Could you check a few things on this model? Use its own coordinates, in mm. Give positions to 0.01 mm unless a question says otherwise; leave off trailing zeros. Order: outer loops, then holes, each group sorted by start corner. A loop starts at its lowest first (then second) coordinate and runs counter-clockwise, first axis right, second up. Notation, with made-up numbers: M 65.25,86.5 L 107.25,86.5 A21 ccw 107.25,111.5 Z; hole C -39.5,22 d10. An arc over 180 degrees is marked long. Use a Markdown table: item, result. Add a question column.
Item 1: If I drill on L1, parallel to Y at x = 45, z = 3.3; L2, parallel to Y at x = 32, z = 4.35; L3, parallel to Y at x = -43.5, z = 3.6, over which ranges is the centre line in solid material (lowest first)? Write a range as from..to.
Item 2: Suppose I cut it at A-A on x = -25.5. Write out the boundary of the cut face in (y, z).
Item 3: Suppose I cut it at B-B on z = 4.2. Write out the boundary of the cut face in (x, y).
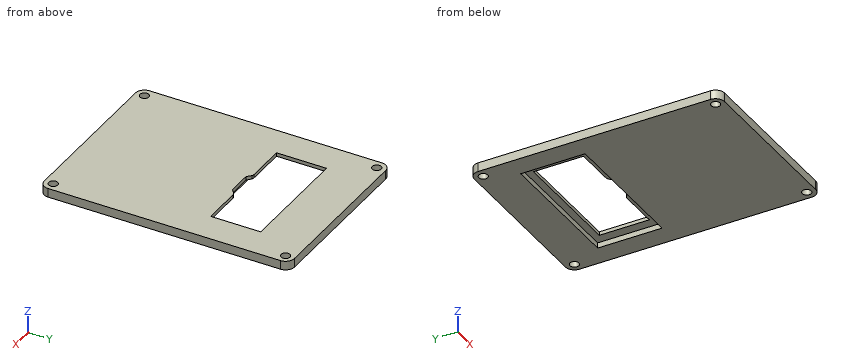
from build123d import *

# Parameters (mm, degrees)
SKETCH1_R           = 2.5
BOSS_EXTRUDE1_DEPTH = 5
CUT_EXTRUDE1_DEPTH  = 5
SKETCH2_4_W         = 76
SKETCH2_4_H         = 36
CUT_EXTRUDE2_DEPTH  = 3


with BuildPart() as part:
    # Sketch1 → Boss-Extrude1 (new body)
    with BuildSketch(Plane.XY):
        with BuildLine():
            Line((-45, 70), (45, 70))
            ThreePointArc((45, 70), (48.535533906, 68.535533906), (50, 65))
            Line((50, 65), (50, -65))
            ThreePointArc((50, -65), (48.535533906, -68.535533906), (45, -70))
            Line((45, -70), (-45, -70))
            ThreePointArc((-45, -70), (-48.535533906, -68.535533906), (-50, -65))
            Line((-50, -65), (-50, 65))
            ThreePointArc((-50, 65), (-48.535533906, 68.535533906), (-45, 70))
        make_face()
        with Locations((-45, 65)):
            Circle(SKETCH1_R, mode=Mode.SUBTRACT)
        with Locations((45, 65)):
            Circle(SKETCH1_R, mode=Mode.SUBTRACT)
        with Locations((45, -65)):
            Circle(SKETCH1_R, mode=Mode.SUBTRACT)
        with Locations((-45, -65)):
            Circle(SKETCH1_R, mode=Mode.SUBTRACT)
    extrude(amount=BOSS_EXTRUDE1_DEPTH)

    # Sketch2 → Cut-Extrude1 (cut)
    with BuildSketch(Plane(origin=(0, 0, 0), x_dir=(-1, 0, 0), z_dir=(0, 0, -1))):
        with BuildLine():
            Line((-8.935788795, 15.50990671), (-6.621919354, 13.5))
            Line((-6.621919354, 13.5), (6.621919354, 13.5))
            Line((6.621919354, 13.5), (8.935788795, 15.50990671))
            ThreePointArc((8.935788795, 15.50990671), (9.547279148, 15.873474502), (10.247345781, 16))
            Line((10.247345781, 16), (32.5, 16))
            Line((32.5, 16), (32.5, 44))
            Line((32.5, 44), (-32.5, 44))
            Line((-32.5, 44), (-32.5, 16))
            Line((-32.5, 16), (-10.247345781, 16))
            ThreePointArc((-10.247345781, 16), (-9.547279148, 15.873474502), (-8.935788795, 15.50990671))
        make_face()
    extrude(amount=-CUT_EXTRUDE1_DEPTH, mode=Mode.SUBTRACT)

    # Sketch2_4 → Cut-Extrude2 (cut)
    with BuildSketch(Plane(origin=(0, 0, 0), x_dir=(-1, 0, 0), z_dir=(0, 0, -1))):
        with Locations((0, 30)):
            Rectangle(SKETCH2_4_W, SKETCH2_4_H)
        with BuildLine():
            Line((-8.935788795, 15.50990671), (-6.621919354, 13.5))
            Line((-6.621919354, 13.5), (6.621919354, 13.5))
            Line((6.621919354, 13.5), (8.935788795, 15.50990671))
            ThreePointArc((8.935788795, 15.50990671), (9.547279148, 15.873474502), (10.247345781, 16))
            Line((10.247345781, 16), (32.5, 16))
            Line((32.5, 16), (32.5, 44))
            Line((32.5, 44), (-32.5, 44))
            Line((-32.5, 44), (-32.5, 16))
            Line((-32.5, 16), (-10.247345781, 16))
            ThreePointArc((-10.247345781, 16), (-9.547279148, 15.873474502), (-8.935788795, 15.50990671))
        make_face(mode=Mode.SUBTRACT)
    extrude(amount=-CUT_EXTRUDE2_DEPTH, mode=Mode.SUBTRACT)


solid = part.part
Findings below:
| question | item | result |
|---|---|---|
| 1 | L1 | y = -70..-67.5, -62.5..62.5, 67.5..70 |
| 1 | L2 | y = -70..16, 44..70 |
| 1 | L3 | y = -70..-67, -63..63, 67..70 |
| 2 | outline | M -70,0 L 12,0 L 12,3 L 16,3 L 16,5 L -70,5 Z; M 44,3 L 48,3 L 48,0 L 70,0 L 70,5 L 44,5 Z |
| 3 | outline | M -50,-65 A5 ccw -45,-70 L 45,-70 A5 ccw 50,-65 L 50,65 A5 ccw 45,70 L -45,70 A5 ccw -50,65 Z; hole C -45,-65 d5; hole C -45,65 d5; hole M -32.5,16 L -10.25,16 A2 cw -8.94,15.51 L -6.62,13.5 L 6.62,13.5 L 8.94,15.51 A2 cw 10.25,16 L 32.5,16 L 32.5,44 L -32.5,44 Z; hole C 45,-65 d5; hole C 45,65 d5 |
